```python
from build123d import *

# Parameters (mm, degrees)
ESQUISSE1_W                  = 287
ESQUISSE1_H                  = 320
BOSS_EXTRU_1_DEPTH           = 1.5
ESQUISSE2_W                  = 23
ESQUISSE2_H                  = 30
ENL_V_MAT_EXTRU_1_DEPTH      = 1
ENL_V_MAT_EXTRU_1_DEPTH_BACK = 2.5
CONG_1_R                     = 10
CONG_2_R                     = 3
ESQUISSE3_W                  = 140
ESQUISSE3_H                  = 92
ENL_V_MAT_EXTRU_2_DEPTH      = 1
ENL_V_MAT_EXTRU_2_DEPTH_BACK = 2.5
ESQUISSE4_W                  = 56.5
ESQUISSE4_H                  = 222
ENL_V_MAT_EXTRU_3_DEPTH      = 1
ENL_V_MAT_EXTRU_3_DEPTH_BACK = 2.5
ESQUISSE5_W                  = 58.5
ESQUISSE5_H                  = 92
ENL_V_MAT_EXTRU_4_DEPTH      = 1
ENL_V_MAT_EXTRU_4_DEPTH_BACK = 2.5
ESQUISSE6_W                  = 146.5
ESQUISSE6_H                  = 16
ENL_V_MAT_EXTRU_5_DEPTH      = 1
ENL_V_MAT_EXTRU_5_DEPTH_BACK = 2.5
CONG_3_R                     = 5
ESQUISSE7_R                  = 2.25
ENL_V_MAT_EXTRU_6_DEPTH      = 1
ENL_V_MAT_EXTRU_6_DEPTH_BACK = 2.5
ESQUISSE8_R                  = 2.25
ENL_V_MAT_EXTRU_7_DEPTH      = 1
ENL_V_MAT_EXTRU_7_DEPTH_BACK = 2.5
ESQUISSE9_W                  = 28
ESQUISSE9_H                  = 15
ENL_V_MAT_EXTRU_8_DEPTH      = 1
ENL_V_MAT_EXTRU_8_DEPTH_BACK = 2.5
CONG_4_R                     = 3
CONG_6_R                     = 2


with BuildPart() as part:
    # Esquisse1 → Boss.-Extru.1 (new body)
    with BuildSketch(Plane.XY):
        with Locations((143.5, 160)):
            Rectangle(ESQUISSE1_W, ESQUISSE1_H)
    extrude(amount=BOSS_EXTRU_1_DEPTH)

    # Esquisse2 → Enlèv. mat.-Extru.1 (cut, two sides)
    with BuildSketch(Plane.XY.offset(1.5)) as enl_v_mat_extru_1_sk:
        with Locations((275.5, 15)):
            Rectangle(ESQUISSE2_W, ESQUISSE2_H)
        with Locations((11.5, 15)):
            Rectangle(ESQUISSE2_W, ESQUISSE2_H)
    extrude(amount=ENL_V_MAT_EXTRU_1_DEPTH, mode=Mode.SUBTRACT)
    extrude(enl_v_mat_extru_1_sk.sketch, amount=-ENL_V_MAT_EXTRU_1_DEPTH_BACK, mode=Mode.SUBTRACT)

    # Congé1
    cong_1_edges = [part.edges().sort_by_distance(p)[0] for p in [
        (264, 30, 0.75),
        (23, 30, 0.75),
    ]]
    fillet(cong_1_edges, radius=CONG_1_R)

    # Congé2
    cong_2_edges = [part.edges().sort_by_distance(p)[0] for p in [
        (287, 30, 0.75),
        (264, 0, 0.75),
        (23, 0, 0.75),
        (0, 30, 0.75),
    ]]
    fillet(cong_2_edges, radius=CONG_2_R)

    # Esquisse3 → Enlèv. mat.-Extru.2 (cut, two sides)
    with BuildSketch(Plane.XY.offset(1.5)) as enl_v_mat_extru_2_sk:
        with Locations((143.5, 274)):
            Rectangle(ESQUISSE3_W, ESQUISSE3_H)
    extrude(amount=ENL_V_MAT_EXTRU_2_DEPTH, mode=Mode.SUBTRACT)
    extrude(enl_v_mat_extru_2_sk.sketch, amount=-ENL_V_MAT_EXTRU_2_DEPTH_BACK, mode=Mode.SUBTRACT)

    # Esquisse4 → Enlèv. mat.-Extru.3 (cut, two sides)
    with BuildSketch(Plane.XY.offset(1.5)) as enl_v_mat_extru_3_sk:
        with Locations((241.75, 209)):
            Rectangle(ESQUISSE4_W, ESQUISSE4_H)
    extrude(amount=ENL_V_MAT_EXTRU_3_DEPTH, mode=Mode.SUBTRACT)
    extrude(enl_v_mat_extru_3_sk.sketch, amount=-ENL_V_MAT_EXTRU_3_DEPTH_BACK, mode=Mode.SUBTRACT)

    # Esquisse5 → Enlèv. mat.-Extru.4 (cut, two sides)
    with BuildSketch(Plane.XY.offset(1.5)) as enl_v_mat_extru_4_sk:
        with Locations((44.25, 274)):
            Rectangle(ESQUISSE5_W, ESQUISSE5_H)
    extrude(amount=ENL_V_MAT_EXTRU_4_DEPTH, mode=Mode.SUBTRACT)
    extrude(enl_v_mat_extru_4_sk.sketch, amount=-ENL_V_MAT_EXTRU_4_DEPTH_BACK, mode=Mode.SUBTRACT)

    # Esquisse6 → Enlèv. mat.-Extru.5 (cut, two sides)
    with BuildSketch(Plane.XY.offset(1.5)) as enl_v_mat_extru_5_sk:
        with Locations((140.25, 106)):
            Rectangle(ESQUISSE6_W, ESQUISSE6_H)
    extrude(amount=ENL_V_MAT_EXTRU_5_DEPTH, mode=Mode.SUBTRACT)
    extrude(enl_v_mat_extru_5_sk.sketch, amount=-ENL_V_MAT_EXTRU_5_DEPTH_BACK, mode=Mode.SUBTRACT)

    # Congé3
    cong_3_edges = [part.edges().sort_by_distance(p)[0] for p in [
        (270, 98, 0.75),
        (15, 228, 0.75),
        (67, 98, 0.75),
        (213.5, 114, 0.75),
        (67, 114, 0.75),
        (213.5, 228, 0.75),
    ]]
    fillet(cong_3_edges, radius=CONG_3_R)

    # Esquisse7 → Enlèv. mat.-Extru.6 (cut, two sides)
    with BuildSketch(Plane.XY.offset(1.5)) as enl_v_mat_extru_6_sk:
        with Locations((277, 300)):
            Circle(ESQUISSE7_R)
        with Locations((277, 270)):
            Circle(ESQUISSE7_R)
        with Locations((10, 270)):
            Circle(ESQUISSE7_R)
        with Locations((10, 300)):
            Circle(ESQUISSE7_R)
        with Locations((277, 83)):
            Circle(ESQUISSE7_R)
        with Locations((277, 53)):
            Circle(ESQUISSE7_R)
        with Locations((10, 53)):
            Circle(ESQUISSE7_R)
        with Locations((10, 83)):
            Circle(ESQUISSE7_R)
        with Locations((33, 170)):
            Circle(ESQUISSE7_R)
        with Locations((103, 170)):
            Circle(ESQUISSE7_R)
        with Locations((173, 170)):
            Circle(ESQUISSE7_R)
    extrude(amount=ENL_V_MAT_EXTRU_6_DEPTH, mode=Mode.SUBTRACT)
    extrude(enl_v_mat_extru_6_sk.sketch, amount=-ENL_V_MAT_EXTRU_6_DEPTH_BACK, mode=Mode.SUBTRACT)

    # Esquisse8 → Enlèv. mat.-Extru.7 (cut, two sides)
    with BuildSketch(Plane.XY.offset(1.5)) as enl_v_mat_extru_7_sk:
        with Locations((133.5, 193)):
            Circle(ESQUISSE8_R)
        with Locations((153.5, 193)):
            Circle(ESQUISSE8_R)
        with Locations((182.5, 193)):
            Circle(ESQUISSE8_R)
        with Locations((202.5, 193)):
            Circle(ESQUISSE8_R)
        with Locations((84.5, 193)):
            Circle(ESQUISSE8_R)
        with Locations((104.5, 193)):
            Circle(ESQUISSE8_R)
    extrude(amount=ENL_V_MAT_EXTRU_7_DEPTH, mode=Mode.SUBTRACT)
    extrude(enl_v_mat_extru_7_sk.sketch, amount=-ENL_V_MAT_EXTRU_7_DEPTH_BACK, mode=Mode.SUBTRACT)

    # Esquisse9 → Enlèv. mat.-Extru.8 (cut, two sides)
    with BuildSketch(Plane.XY.offset(1.5)) as enl_v_mat_extru_8_sk:
        with Locations((143.5, 207.5)):
            Rectangle(ESQUISSE9_W, ESQUISSE9_H)
        with Locations((196, 207.5)):
            Rectangle(ESQUISSE9_W, ESQUISSE9_H)
        with Locations((91, 207.5)):
            Rectangle(ESQUISSE9_W, ESQUISSE9_H)
    extrude(amount=ENL_V_MAT_EXTRU_8_DEPTH, mode=Mode.SUBTRACT)
    extrude(enl_v_mat_extru_8_sk.sketch, amount=-ENL_V_MAT_EXTRU_8_DEPTH_BACK, mode=Mode.SUBTRACT)

    # Congé4
    cong_4_edges = [part.edges().sort_by_distance(p)[0] for p in [
        (129.5, 200, 0.75),
        (129.5, 215, 0.75),
        (157.5, 215, 0.75),
        (157.5, 200, 0.75),
        (182, 215, 0.75),
        (210, 215, 0.75),
        (210, 200, 0.75),
        (182, 200, 0.75),
        (77, 200, 0.75),
        (77, 215, 0.75),
        (105, 215, 0.75),
        (105, 200, 0.75),
    ]]
    fillet(cong_4_edges, radius=CONG_4_R)

    # Congé6
    cong_6_edges = [part.edges().sort_by_distance(p)[0] for p in [
        (270, 320, 0.75),
        (15, 320, 0.75),
        (0, 320, 0.75),
        (287, 320, 0.75),
    ]]
    fillet(cong_6_edges, radius=CONG_6_R)


solid = part.part
```
Check sheet for the modelled part. Datum: model origin and axes. Units: mm. Give positions to 0.01 mm unless a question says otherwise; leave off trailing zeros. Order: outer loops, then holes, each group sorted by start corner. A loop starts at its lowest first (then second) coordinate and runs counter-clockwise, first axis right, second up. Notation, with made-up numbers: M -10.75,27.5 L -2.75,27.5 A21 ccw -2.75,63.5 Z; hole C 75.5,-34 d4. An arc over 180 degrees is marked long. Answer in a Markdown table with one row per item. Add a question column.
Q1. Sectioned sample at B-B, the plane z = 0.6. Count the separate pieces of the cut face and the enclosed holes in it, and give its area (3 significant figures).
Q2. Gauge pin test, flat ends, axial feed: pin 1 Ø5 at (x, y) = (173, 170) entering from -Z; pin 2 Ø0.8 at (x, z) = (145.5, 1) entering from +Y; pin 3 Ø0.8 at (y, z) = (10.5, 0.5) entering from -X; pin 4 Ø2.5 at (x, y) = (277, 270) entering from -Z. Record the tip position at first contact, or that the pin passes through.
Q3. Sectioned sample at A-A, the plane x = 141. Record the boundary of the cut face in (y, z), and give its area (4 significant figures).
Q4. Thickness scan on L1, parallel to Y at x = 145.5, z = 1.25; L2, parallel to Y at x = 10, z = 0.4; L3, parallel to X at y = 270, z = 0.35. Record the ranges inside material, lowest first.
Q5. Sectioned sample at C-C, the plane x = 249. Record the boundary of the cut face in (y, z).
Verdict:
| question | item | result |
|---|---|---|
| 1 | separate pieces | 1 |
| 1 | enclosed holes | 20 |
| 1 | area | 55,800 mm² |
| 2 | pin 1 | z = 0 |
| 2 | pin 2 | y = 228 |
| 2 | pin 3 | x = 23 |
| 2 | pin 4 | through |
| 3 | outline | M 0,0 L 98,0 L 98,1.5 L 0,1.5 Z; M 114,0 L 200,0 L 200,1.5 L 114,1.5 Z; M 215,0 L 228,0 L 228,1.5 L 215,1.5 Z |
| 3 | area | 295.5 mm² |
| 4 | L1 | 0 to 98, 114 to 200, 215 to 228 |
| 4 | L2 | 30 to 50.75, 55.25 to 80.75, 85.25 to 267.75, 272.25 to 297.75, 302.25 to 320 |
| 4 | L3 | 0 to 7.75, 12.25 to 15, 270 to 274.75, 279.25 to 287 |
| 5 | outline | M 0,0 L 98,0 L 98,1.5 L 0,1.5 Z |
